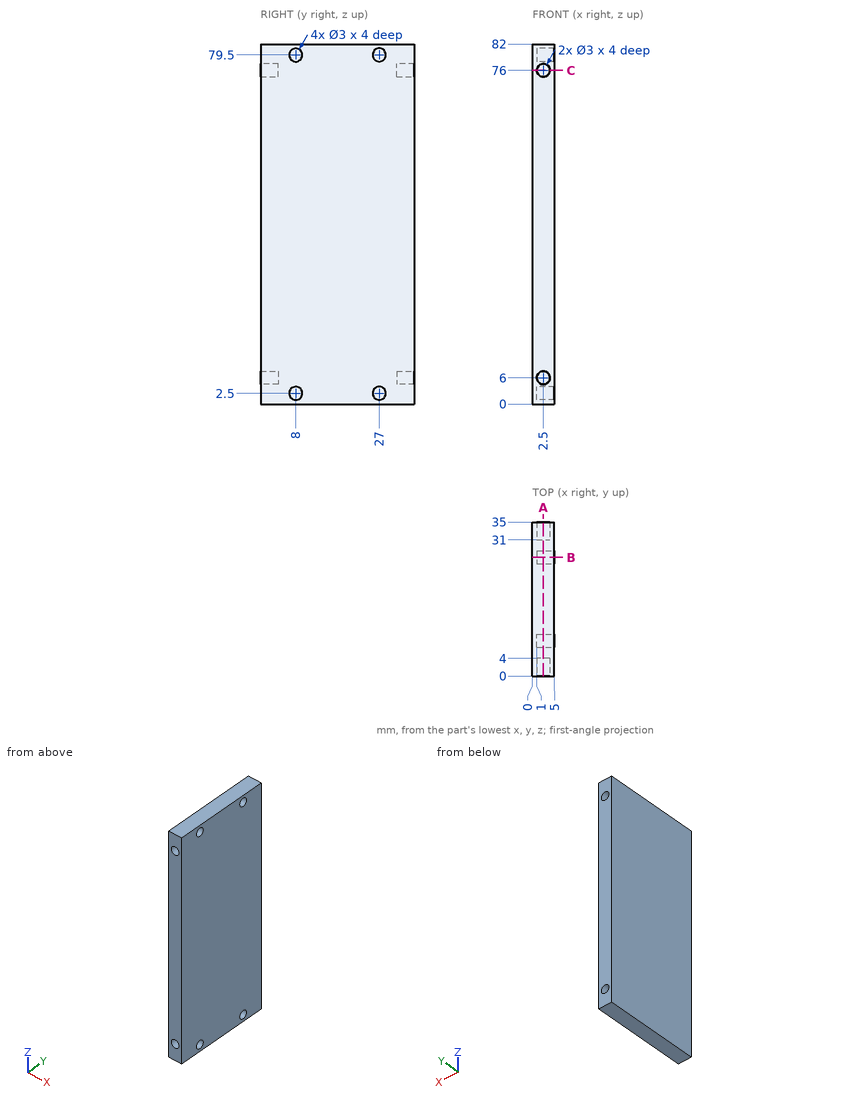
Could you check a few things on this drawing? It's one solid part, dimensions in mm from its lowest x, y, z. Round coordinates to 2 decimals unless told otherwise and drop trailing zeros. Order: outer loops, then holes, each group sorted by start corner. A loop starts at its lowest first (then second) coordinate and runs counter-clockwise, first axis right, second up.
(1) I'm going to push flat-ended pins straight in: pin 1 (1.8 mm diameter, centred on y = 8, z = 79.5, fed in from +X); pin 2 (2.5 mm diameter, centred on x = 2.5, z = 76, fed in from +Y); pin 3 (1.5 mm diameter, centred on x = 2.5, z = 5.5, fed in from -Y). Where does each tip first touch, or does it pass through?
Response values:
pin 1: stops at x = 1
pin 2: stops at y = 31
pin 3: stops at y = 4
(2) Imagine slicing it at A-A (x = 2.5). Write out the boundary of the cut face in (y, z).
Response values:
outline: (0, 0) - (35, 0) - (35, 4.5) - (31, 4.5) - (31, 7.5) - (35, 7.5) - (35, 74.5) - (31, 74.5) - (31, 77.5) - (35, 77.5) - (35, 82) - (0, 82) - (0, 77.5) - (4, 77.5) - (4, 74.5) - (0, 74.5) - (0, 7.5) - (4, 7.5) - (4, 4.5) - (0, 4.5) - close; hole circle Ø3 at (8, 2.5); hole circle Ø3 at (8, 79.5); hole circle Ø3 at (27, 2.5); hole circle Ø3 at (27, 79.5)
(3) Imagine slicing it at C-C (z = 76). Write out the boundary of the cut face in (x, y).
Response values:
outline: (0, 0) - (1, 0) - (1, 4) - (4, 4) - (4, 0) - (5, 0) - (5, 35) - (4, 35) - (4, 31) - (1, 31) - (1, 35) - (0, 35) - close
(4) Imagine slicing it at B-B (y = 27). Write out the boundary of the cut face in (x, z).
Response values:
outline: (0, 0) - (5, 0) - (5, 1) - (1, 1) - (1, 4) - (5, 4) - (5, 78) - (1, 78) - (1, 81) - (5, 81) - (5, 82) - (0, 82) - close
(5) Please list where these lines run through material, in increasing order: line 1 along Y through (x, z) = (1.95, 79.5); line 2 along Z through (x, y) = (3.8, 7.5); line 3 along Y through (x, z) = (4.65, 3).
Response values:
line 1: y = 0 to 6.5, 9.5 to 25.5, 28.5 to 35
line 2: z = 0 to 1.09, 3.91 to 78.09, 80.91 to 82
line 3: y = 0 to 6.59, 9.41 to 25.59, 28.41 to 35
